from build123d import *

# Parameters (mm, degrees)
F0_W     = 81.7074924707
F0_H     = 82.3852196336
F0_R     = 22.0154906443
F1_DEPTH = 34.544
F0_R_2   = 12.2186254277
F2_DEPTH = 52.07
F3_DEPTH = 147


# Not quite as in the source:
# - an extrude ends at something that could not be found from the text; its depth is read off the source's solid


with BuildPart() as f1:
    # F0 (on Front) → F1 (new body)
    with BuildSketch(Plane.XZ):
        Rectangle(F0_W, F0_H)
        Circle(F0_R, mode=Mode.SUBTRACT)
    extrude(amount=F1_DEPTH)

    # F0 (on Front) → F2 (join)
    with BuildSketch(Plane.XZ):
        Circle(F0_R)
        Circle(F0_R_2, mode=Mode.SUBTRACT)
    extrude(amount=F2_DEPTH)

    # F0 (on Front) → F3 (cut, through all)
    with BuildSketch(Plane.XZ):
        Circle(F0_R_2)
    extrude(amount=-F3_DEPTH, mode=Mode.SUBTRACT)


solid = f1.part
Can you work these out from the model? Positions are in its coordinate system, mm. A direction names the side the tool comes from. Coordinates: 2 decimals unless noted, no trailing zeros. Write each loop counter-clockwise with the first axis right and the second up, starting at its lowest first coordinate (ties: lowest second). Pieces come first, ordered by that corner, then holes. Notation, with made-up numbers: (86, -35) - (102, -35) arc R16 cw to (102, -20) - close; hole circle Ø5 at (-13, 53.5). An arc over 180 degrees is marked (long way). Return JSON: item names as keys, results as strings. Group by question number.
Item 1: We'd pull the mould along Z, two halves only. Please class faces 3 (the face through (-2.649, -25.671, -11.928)), 4 (the face through (-40.854, -17, -1)), 5 (the face through (-1, -17, -41.193)): pulls with the +Z half, pulls with the -Z half, needs draft (parallel to the pull), parting line crosses it, or undercut.
Item 2: Please list where these lines run through material, in increasing order: probe 1 along Z at (x, y) = (0, -14); probe 2 along Z at (x, y) = (0, -38); probe 3 along Y at (x, z) = (15, -35.5).
Item 3: I'm going to push a flat-ended pin straight in: pin 1 Ø6 at (x, y) = (14.5, -42.5) entering from +Z. Where does the tip first touch, or does it pass through?
Item 4: If we section it at D-D (z = 14): Write out the boundary of the cut face in (x, y).
Item 5: If we section it at A-A (z = 0): Write out the boundary of the cut face in (x, y).
Item 6: Which directions (+Z, -Z, +X, -X, +Y, -Y) give clear straight access to the entire face, cutting with the end or side of a thin tool? Please do faces 1 (the face through (21, -43.18, 6.61)), 2 (the face through (9, -52.07, -9)).
Item 7: If we section it at C-C (y = -8): Write out the boundary of the cut face in (x, z), then the cut area to 3 significant figures.
Item 8: If we section it at B-B (x = 0): Write out the boundary of the cut face in (y, z).
Return value:
{
 "1": {"face 3": "undercut", "face 4": "needs draft", "face 5": "pulls with the -Z half"},
 "2": {"probe 1": "z = -41.19 to -12.22, 12.22 to 41.19", "probe 2": "z = -22.02 to -12.22, 12.22 to 22.02", "probe 3": "y = -34.54 to 0"},
 "3": {"pin 1": "stops at z = 18.77"},
 "4": {"outline": "(-40.85, -34.54) - (-16.99, -34.54) - (-16.99, -52.07) - (16.99, -52.07) - (16.99, -34.54) - (40.85, -34.54) - (40.85, 0) - (-40.85, 0) - close"},
 "5": {"outline": "(-40.85, -34.54) - (-22.02, -34.54) - (-22.02, -52.07) - (-12.22, -52.07) - (-12.22, 0) - (-40.85, 0) - close; (12.22, -52.07) - (22.02, -52.07) - (22.02, -34.54) - (40.85, -34.54) - (40.85, 0) - (12.22, 0) - close"},
 "6": {"face 1": "-Y", "face 2": "+Z, -Z, +X, -X, -Y"},
 "7": {"outline": "(-40.85, -41.19) - (40.85, -41.19) - (40.85, 41.19) - (-40.85, 41.19) - close; hole circle Ø24.44 at (0, 0)", "area": "6,260 mm^2"},
 "8": {"outline": "(-52.07, -22.02) - (-34.54, -22.02) - (-34.54, -41.19) - (0, -41.19) - (0, -12.22) - (-52.07, -12.22) - close; (-52.07, 12.22) - (0, 12.22) - (0, 41.19) - (-34.54, 41.19) - (-34.54, 22.02) - (-52.07, 22.02) - close"}
}
